```python
from build123d import *

# Parameters (mm, degrees)
BOSS_EXTRUDE2_DEPTH      = 5.3
SKETCH2_R                = 0.5
BOSS_EXTRUDE3_DEPTH      = 5.3
BOSS_EXTRUDE3_DEPTH_BACK = 1
FILLET2_R                = 0.5
SKETCH4_W                = 5
SKETCH4_H                = 48
CUT_EXTRUDE1_DEPTH       = 0.3


with BuildPart() as part:
    # Sketch1 → Boss-Extrude2 (new body)
    with BuildSketch(Plane(origin=(0, 0, 0), x_dir=(1, 0, 0), z_dir=(0, 1, 0))):
        with BuildLine():
            Line((-34.5, -24.5), (34.5, -24.5))
            ThreePointArc((34.5, -24.5), (34.853553391, -24.353553391), (35, -24))
            Line((35, -24), (35, 24))
            ThreePointArc((35, 24), (34.853553391, 24.353553391), (34.5, 24.5))
            Line((34.5, 24.5), (-34.5, 24.5))
            ThreePointArc((-34.5, 24.5), (-34.853553391, 24.353553391), (-35, 24))
            Line((-35, 24), (-35, -24))
            ThreePointArc((-35, -24), (-34.853553391, -24.353553391), (-34.5, -24.5))
        make_face()
    extrude(amount=BOSS_EXTRUDE2_DEPTH)

    # Sketch2 → Boss-Extrude3 (add, two sides)
    with BuildSketch(Plane.XY.offset(24.5)) as boss_extrude3_sk:
        with Locations((-34.3, 1.279563796)):
            Circle(SKETCH2_R)
        with Locations((-34.3, 4.020436204)):
            Circle(SKETCH2_R)
    extrude(amount=BOSS_EXTRUDE3_DEPTH)
    extrude(boss_extrude3_sk.sketch, amount=-BOSS_EXTRUDE3_DEPTH_BACK)

    # Fillet2
    fillet2_edges = [part.edges().sort_by_distance(p)[0] for p in [
        (34.853553391, 5.3, 24.353553391),
        (0, 0, 24.5),
        (-34.853553391, 0, 24.353553391),
        (35, 5.3, 0),
        (34.853553391, 5.3, -24.353553391),
        (0, 5.3, -24.5),
        (-34.853553391, 5.3, -24.353553391),
        (-35, 5.3, 0),
        (-34.853553391, 5.3, 24.353553391),
        (0, 5.3, 24.5),
        (-35, 0, 0),
        (-34.853553391, 0, -24.353553391),
        (0, 0, -24.5),
        (34.853553391, 0, -24.353553391),
        (35, 0, 0),
        (34.853553391, 0, 24.353553391),
    ]]
    fillet(fillet2_edges, radius=FILLET2_R)

    # Sketch4 → Cut-Extrude1 (cut)
    with BuildSketch(Plane(origin=(0, 5.3, 0), x_dir=(1, 0, 0), z_dir=(0, 1, 0))):
        with Locations((-32, 0)):
            Rectangle(SKETCH4_W, SKETCH4_H)
    extrude(amount=-CUT_EXTRUDE1_DEPTH, mode=Mode.SUBTRACT)


solid = part.part
```
Geometry check sheet. Reference: the model listing, model coordinates, mm. Coordinates: 2 decimals unless noted, no trailing zeros. Order: outer loops, then holes, each group sorted by start corner. A loop starts at its lowest first (then second) coordinate and runs counter-clockwise, first axis right, second up.
Item 1: Scan line: line 1 along Z through (x, y) = (26, 1.15). Record every from-to range of solid material in increasing order.
Item 2: Mould release check, pull along Z, two halves, no side actions. Record for faces 1 (the flat face through (-32, 5, 0)), 2 (the flat face through (0, 3, 24.5)), 3 (the flat face through (0, 3, -24.5)), 4 (the flat face through (35, 3, 0)): released by +Z, released by -Z, zero draft, split by the parting line, or undercut.
Item 3: Depth check by flat-ended pin: pin 1 (1.3 mm diameter, centred on x = -8, y = 2, fed in from +Z). Enter the tip coordinate at first touch or a pass-through.
Item 4: Section check A-A (x = 26). Enter the section's corners in (y, z).
Check sheet entries:
1. line 1: z = -24.5 to 24.5
2. face 1: undercut
2. face 2: released by +Z
2. face 3: released by -Z
2. face 4: zero draft
3. pin 1: stops at z = 24.5
4. outline: (0, -24) arc R0.5 ccw to (0.5, -24.5) - (4.8, -24.5) arc R0.5 ccw to (5.3, -24) - (5.3, 24) arc R0.5 ccw to (4.8, 24.5) - (0.5, 24.5) arc R0.5 ccw to (0, 24) - close
